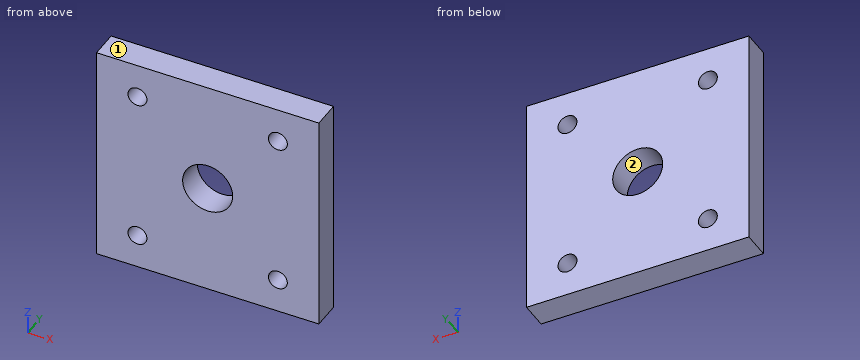
```python
from build123d import *

# Parameters (mm, degrees)
CROQUIS1_W              = 40
CROQUIS1_H              = 40
CROQUIS1_R              = 4.5
SALIENTE_EXTRUIR1_DEPTH = 5
CROQUIS2_R              = 1.7
CORTAR_EXTRUIR1_DEPTH   = 10


with BuildPart() as part:
    # Croquis1 → Saliente-Extruir1 (new body)
    with BuildSketch(Plane(origin=(0, 0, 0), x_dir=(1, 0, 0), z_dir=(0, 1, 0))):
        Rectangle(CROQUIS1_W, CROQUIS1_H)
        Circle(CROQUIS1_R, mode=Mode.SUBTRACT)
    extrude(amount=SALIENTE_EXTRUIR1_DEPTH)

    # Croquis2 → Cortar-Extruir1 (cut)
    with BuildSketch(Plane.XZ):
        with Locations((12.628756813, -13.795283125)):
            Circle(CROQUIS2_R)
        with Locations((12.628756813, 13.795283125)):
            Circle(CROQUIS2_R)
        with Locations((-12.628756813, 13.795283125)):
            Circle(CROQUIS2_R)
        with Locations((-12.628756813, -13.795283125)):
            Circle(CROQUIS2_R)
    extrude(amount=-CORTAR_EXTRUIR1_DEPTH, mode=Mode.SUBTRACT)


solid = part.part
```
Check sheet for the modelled part. Datum: model origin and axes. Units: mm. Face numbers are marked on the shaded views. Coordinates: 2 decimals unless noted, no trailing zeros. Order: outer loops, then holes, each group sorted by start corner. A loop starts at its lowest first (then second) coordinate and runs counter-clockwise, first axis right, second up. Notation, with made-up numbers: (-21.5, 6) -> (2.5, 6) arc R24 ccw to (2.5, 27) -> close; hole circle Ø4 at (23, -11). An arc over 180 degrees is marked (long way). Write each question's results on one line, items separated by ' | '. Start each with the question number.
1) Section check A-A (z = 0). Enter the section's corners in (x, y).
2) Section check B-B (x = 0). Enter the section's corners in (y, z), and give its area (3 significant figures).
3) Material ranges on line 1 along Z through (x, y) = (0, 1.1); line 2 along Z through (x, y) = (-13, 2); line 3 along Z through (x, y) = (-12, 3.6), recorded low to high.
4) Draft check along X on the marked faces 1 and 2. Enter one of: pulls with the +X half, pulls with the -X half, needs draft (parallel to the pull), parting line crosses it, or undercut.
5) Depth check by flat-ended pin: pin 1 (5.5 mm diameter, centred on x = 0, z = 0, fed in from -Y) (3 decimals). Enter the tip coordinate at first touch or a pass-through.
6) Section check C-C (y = 3.45). Enter the section's corners in (x, z).
Checked values:
1) outline: (-20, 0) -> (-4.5, 0) -> (-4.5, 5) -> (-20, 5) -> close; (4.5, 0) -> (20, 0) -> (20, 5) -> (4.5, 5) -> close
2) outline: (0, -20) -> (5, -20) -> (5, -4.5) -> (0, -4.5) -> close; (0, 4.5) -> (5, 4.5) -> (5, 20) -> (0, 20) -> close | area: 155 mm²
3) line 1: -20 to -4.5, 4.5 to 20 | line 2: -20 to -15.45, -12.14 to 12.14, 15.45 to 20 | line 3: -20 to -15.37, -12.22 to 12.22, 15.37 to 20
4) face 1: needs draft | face 2: undercut
5) pin 1: through
6) outline: (-20, -20) -> (20, -20) -> (20, 20) -> (-20, 20) -> close; hole circle Ø3.4 at (-12.63, -13.8); hole circle Ø3.4 at (-12.63, 13.8); hole circle Ø9 at (0, 0); hole circle Ø3.4 at (12.63, -13.8); hole circle Ø3.4 at (12.63, 13.8)
